Could you check a few things on this model? Use its own coordinates, in mm. Face numbers are marked on the shaded views. A direction names the side the tool comes from. Give positions to 0.01 mm unless a question says otherwise; leave off trailing zeros. Write each loop counter-clockwise with the first axis right and the second up, starting at its lowest first coordinate (ties: lowest second). Pieces come first, ordered by that corner, then holes. Notation, with made-up numbers: (-23.75, 47) - (24.25, 47) arc R16 ccw to (24.25, 73) - close; hole circle Ø4 at (60.5, 11.25). An arc over 180 degrees is marked (long way). Answer as a JSON object with one key per item and string values. Group by question number.
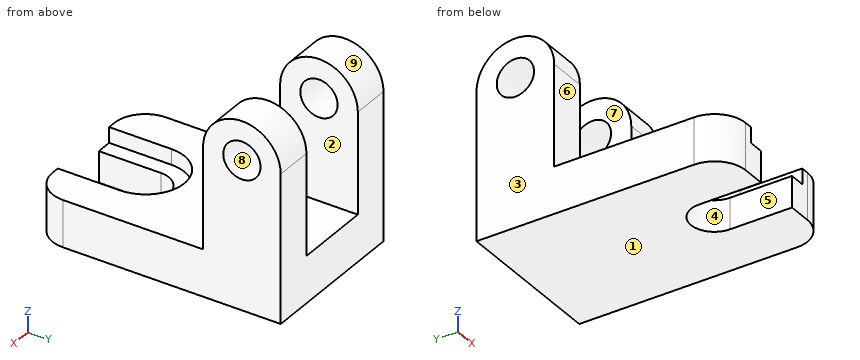
```python
from build123d import *

# Parameters (mm, degrees)
F1_DEPTH = 25
F2_DEPTH = 12.5
F3_R     = 10
F4_W     = 15
F4_H     = 5
F5_DEPTH = 15
F4_W_2   = 5
F6_DEPTH = 5


with BuildPart() as f1:
    # F0 (on Right) → F1 (new body, symmetric)
    with BuildSketch(Plane.YZ):
        Polygon((-80, 0), (0, 0), (0, 15), (-25, 15), (-80, 15), align=None)
        with BuildLine():
            Line((-25, 15), (0, 15))
            Line((0, 15), (0, 47.5))
            ThreePointArc((0, 47.5), (-12.5, 35), (-25, 47.5))
            Line((-25, 47.5), (-25, 15))
        make_face()
        with BuildLine():
            ThreePointArc((-25, 47.5), (-12.5, 35), (0, 47.5))
            Line((0, 47.5), (-6.5, 47.5))
            ThreePointArc((-6.5, 47.5), (-12.5, 41.5), (-18.5, 47.5))
            Line((-18.5, 47.5), (-25, 47.5))
        make_face()
        with BuildLine():
            Line((-6.5, 47.5), (0, 47.5))
            ThreePointArc((0, 47.5), (-12.5, 60), (-25, 47.5))
            Line((-25, 47.5), (-18.5, 47.5))
            ThreePointArc((-18.5, 47.5), (-12.5, 53.5), (-6.5, 47.5))
        make_face()
    extrude(amount=F1_DEPTH, both=True)

    # F0 (on Right) → F2 (cut, symmetric)
    with BuildSketch(Plane.YZ):
        with BuildLine():
            Line((-25, 15), (0, 15))
            Line((0, 15), (0, 47.5))
            ThreePointArc((0, 47.5), (-12.5, 35), (-25, 47.5))
            Line((-25, 47.5), (-25, 15))
        make_face()
        with BuildLine():
            ThreePointArc((-25, 47.5), (-12.5, 35), (0, 47.5))
            Line((0, 47.5), (-6.5, 47.5))
            ThreePointArc((-6.5, 47.5), (-12.5, 41.5), (-18.5, 47.5))
            Line((-18.5, 47.5), (-25, 47.5))
        make_face()
        with BuildLine():
            ThreePointArc((-18.5, 47.5), (-12.5, 41.5), (-6.5, 47.5))
            Line((-6.5, 47.5), (-18.5, 47.5))
        make_face()
        with BuildLine():
            Line((-18.5, 47.5), (-6.5, 47.5))
            ThreePointArc((-6.5, 47.5), (-12.5, 53.5), (-18.5, 47.5))
        make_face()
        with BuildLine():
            Line((-6.5, 47.5), (0, 47.5))
            ThreePointArc((0, 47.5), (-12.5, 60), (-25, 47.5))
            Line((-25, 47.5), (-18.5, 47.5))
            ThreePointArc((-18.5, 47.5), (-12.5, 53.5), (-6.5, 47.5))
        make_face()
    extrude(amount=F2_DEPTH, both=True, mode=Mode.SUBTRACT)

    # F3
    f3_edges = [f1.edges().sort_by_distance(p)[0] for p in [
        (25, -80, 7.5),
        (-25, -80, 7.5),
    ]]
    fillet(f3_edges, radius=F3_R)

    # F4 (on face) → F5 (cut, through all)
    with BuildSketch(Plane.XY.offset(15)):
        with BuildLine():
            Line((-7.5, -60), (-7.5, -75))
            Line((-7.5, -75), (7.5, -75))
            Line((7.5, -75), (7.5, -60))
            ThreePointArc((7.5, -60), (0, -52.5), (-7.5, -60))
        make_face()
        with Locations((0, -77.5)):
            Rectangle(F4_W, F4_H)
    extrude(amount=-F5_DEPTH, mode=Mode.SUBTRACT)

    # F4 (on face) → F6 (cut)
    with BuildSketch(Plane.XY.offset(15)):
        with BuildLine():
            Line((-12.5, -75), (-7.5, -75))
            Line((-7.5, -75), (-7.5, -60))
            ThreePointArc((-7.5, -60), (0, -52.5), (7.5, -60))
            Line((7.5, -60), (7.5, -75))
            Line((7.5, -75), (12.5, -75))
            Line((12.5, -75), (12.5, -60))
            ThreePointArc((12.5, -60), (0, -47.5), (-12.5, -60))
            Line((-12.5, -60), (-12.5, -75))
        make_face()
        with Locations((-10, -77.5)):
            Rectangle(F4_W_2, F4_H)
        with Locations((10, -77.5)):
            Rectangle(F4_W_2, F4_H)
    extrude(amount=-F6_DEPTH, mode=Mode.SUBTRACT)


solid = f1.part
```
(1) I want a section at D-D, the plane x = 10. Please give me the cut outline in (y, z), and give its area (3 significant figures).
(2) Will these pins go through, and if not, where does the flat tip stop? P1, Ø14, axis at x = 20.5, z = 35, coming from the -Y side; P2, Ø8, axis at y = -72.5, z = 7.5, coming from the -X side; P3, Ø9.5, axis at y = -12.5, z = 47.5, coming from the -X side; P4, Ø25, axis at x = 12.5, y = -52, coming from the +Z side.
(3) I want a section at A-A, the plane z = 31.5. Please give me the cut outline in (x, y).
(4) If we mould it in two halves opening along X, with no side actions, what happens to the marked faces 1, 2, 3 and 4? For each: +X half, -X half, draft (parallel to the pull), parting line (faces both ways), or undercut.
(5) For the marked faces 5, 6, 7, 8 and 9, which set-ups out of +Z, -Z, +X, -X, +Y, -Y let a thin tool reach every point of the face, with its end or its side?
(6) I want a section at C-C, the plane x = 19. Please give me the cut outline in (y, z).
(7) I need wall thicknesses on L1, parallel to Y at x = -17, z = 47.5; L2, parallel to Z at x = 18, y = -12; L3, parallel to X at y = -14, z = 34.5. Which ranges of each line are inside material? Lowest first, please.
(8) I want a section at B-B, the plane y = -12.5. Please give me the cut outline in (x, z), and give its area (4 significant figures).
Entries:
{
 "1": {"outline": "(-80, 0) - (0, 0) - (0, 15) - (-52.5, 15) - (-52.5, 10) - (-80, 10) - close", "area": "1,060 mm^2"},
 "2": {"P1": "y = -25", "P2": "x = -25", "P3": "through", "P4": "z = 15"},
 "3": {"outline": "(-25, -25) - (-12.5, -25) - (-12.5, 0) - (-25, 0) - close; (12.5, -25) - (25, -25) - (25, 0) - (12.5, 0) - close"},
 "4": {"face 1": "draft", "face 2": "undercut", "face 3": "-X half", "face 4": "undercut"},
 "5": {"face 5": "+Z, -Z, -Y", "face 6": "+Z, +X, -X, -Y", "face 7": "+Z, +Y, -Y", "face 8": "+X, -X", "face 9": "+Z, +X, -X"},
 "6": {"outline": "(-79.17, 0) - (0, 0) - (0, 47.5) arc R12.5 ccw to (-25, 47.5) - (-25, 15) - (-79.17, 15) - close; hole circle Ø12 at (-12.5, 47.5)"},
 "7": {"L1": "-25 to -18.5, -6.5 to 0", "L2": "0 to 41.52, 53.48 to 59.99", "L3": "-25 to -12.5, 12.5 to 25"},
 "8": {"outline": "(-25, 0) - (25, 0) - (25, 41.5) - (12.5, 41.5) - (12.5, 15) - (-12.5, 15) - (-12.5, 41.5) - (-25, 41.5) - close; (-25, 53.5) - (-12.5, 53.5) - (-12.5, 60) - (-25, 60) - close; (12.5, 53.5) - (25, 53.5) - (25, 60) - (12.5, 60) - close", "area": "1,575 mm^2"}
}
